from build123d import *

# Parameters (mm, degrees)
PAD015_DEPTH       = 15
SKETCH034_R        = 2
POCKET016_DEPTH    = 9.501
SKETCH_W           = 19.6
SKETCH_H           = 18.5
SKETCH_R           = 7.6
PAD_DEPTH          = 22
SKETCH002_W        = 17.1
SKETCH002_H        = 8.4
PAD001_DEPTH       = 8.5
POCKET_DEPTH       = 8
PAD002_DEPTH       = 13.6
SKETCH005_R        = 2
POCKET001_DEPTH    = 22.001
POCKET002_DEPTH    = 101.929968
POLARPATTERN_COUNT = 8
PAD004_DEPTH       = 1.5
SKETCH041_R        = 1.3
POCKET020_DEPTH    = 5


with BuildPart() as body026:
    # Sketch033 (on DatumPlane) → Pad015 (new body)
    with BuildSketch(Plane(origin=(0, -9.8, 0), x_dir=(0, 0, 1), z_dir=(0, -1, 0))):
        with BuildLine():
            Line((-9.5, 0), (-0.25, 0))
            Line((-0.25, 0), (-0.25, 6.907629))
            ThreePointArc((-0.25, 15.092371), (-4.1, 11), (-0.25, 6.907629))
            Line((-0.25, 15.092371), (-0.25, 22))
            Line((-0.25, 22), (-9.5, 22))
            Line((-9.5, 22), (-9.5, 0))
        make_face()
    extrude(amount=PAD015_DEPTH)

    # Sketch034 → Pocket016 (cut, through all)
    with BuildSketch(Plane.XY):
        with Locations((-18.546185, -13.8)):
            Circle(SKETCH034_R)
        with Locations((-3.453815, -13.8)):
            Circle(SKETCH034_R)
        with Locations((-3.453815, -20.8)):
            Circle(SKETCH034_R)
        with Locations((-18.546185, -20.8)):
            Circle(SKETCH034_R)
    extrude(amount=-POCKET016_DEPTH, mode=Mode.SUBTRACT)


with BuildPart() as printable_axisholder_y_fusion:
    # Sketch → Pad (new body)
    with BuildSketch(Plane.YZ):
        with Locations((0, -0.25)):
            Rectangle(SKETCH_W, SKETCH_H)
        Circle(SKETCH_R, mode=Mode.SUBTRACT)
    extrude(amount=-PAD_DEPTH)

    # Sketch002 → Pad001 (join)
    with BuildSketch(Plane(origin=(0, 0, 9), x_dir=(0, -1, 0), z_dir=(0, 0, 1))):
        with Locations((-1.25, -17.8)):
            Rectangle(SKETCH002_W, SKETCH002_H)
    extrude(amount=PAD001_DEPTH)

    # Sketch003 → Pocket (cut)
    with BuildSketch(Plane(origin=(0, -7.3, 0), x_dir=(0, 0, -1), z_dir=(0, -1, 0))):
        with BuildLine():
            Line((-10.5, -22), (-10.5, -13.6))
            Line((-10.5, -13.6), (-11.6, -13.6))
            ThreePointArc((-12.1, -14.1), (-11.746447, -13.953553), (-11.6, -13.6))
            ThreePointArc((-12.1, -14.1), (-12.6, -14.6), (-12.1, -15.1))
            ThreePointArc((-12.1, -16.1), (-11.6, -15.6), (-12.1, -15.1))
            ThreePointArc((-12.1, -16.1), (-12.6, -16.6), (-12.1, -17.1))
            ThreePointArc((-12.1, -18.1), (-11.6, -17.6), (-12.1, -17.1))
            ThreePointArc((-12.1, -18.1), (-12.6, -18.6), (-12.1, -19.1))
            ThreePointArc((-12.1, -20.1), (-11.6, -19.6), (-12.1, -19.1))
            ThreePointArc((-12.1, -20.1), (-12.6, -20.6), (-12.1, -21.1))
            ThreePointArc((-11.8, -22), (-11.625658, -21.441886), (-12.1, -21.1))
            Line((-11.8, -22), (-10.5, -22))
        make_face()
    extrude(amount=-POCKET_DEPTH, mode=Mode.SUBTRACT)

    # Sketch004 (on DatumPlane) → Pad002 (join)
    with BuildSketch(Plane.YZ):
        Polygon((9.8, 17.5), (1.3, 17.5), (1.3, 16.25), (8.55, 16.25), (8.55, 9), (9.8, 9), align=None)
    extrude(amount=-PAD002_DEPTH)

    # Sketch005 (on DatumPlane) → Pocket001 (cut, through all)
    with BuildSketch(Plane.YZ):
        with Locations((4, 12.625)):
            Circle(SKETCH005_R)
    extrude(amount=-POCKET001_DEPTH, mode=Mode.SUBTRACT)

    # Sketch006 (on DatumPlane) → Pocket002 (cut, through all)
    with BuildSketch(Plane.YZ):
        with BuildLine():
            ThreePointArc((-7.846282, 1.560723), (-8, 0), (-7.846282, -1.560723))
            Line((-6.708571, -1.334418), (-7.846282, -1.560723))
            ThreePointArc((-6.708571, 1.334418), (-6.84, 0), (-6.708571, -1.334418))
            Line((-6.708571, 1.334418), (-7.846282, 1.560723))
        make_face()
    pocket002 = extrude(amount=-POCKET002_DEPTH, mode=Mode.SUBTRACT)

    # PolarPattern: Pocket002 ×8 about axis
    polarpattern_axis = Axis((0, 0, 0), (1, 0, 0))
    for i in range(1, POLARPATTERN_COUNT):
        add(pocket002.rotate(polarpattern_axis, i * 360 / POLARPATTERN_COUNT), mode=Mode.SUBTRACT)

    # Sketch010 (on DatumPlane) → Pad004 (join)
    with BuildSketch(Plane.XY.offset(9)):
        Polygon((0, -7.8), (-13.6, -7.8), (-13.6, -7.3), (-22, -7.3), (-22, -9.8), (0, -9.8), align=None)
    extrude(amount=PAD004_DEPTH)

    # Sketch041 → Pocket020 (cut)
    with BuildSketch(Plane.XY.offset(-9.5)):
        with Locations((-11, 0)):
            Circle(SKETCH041_R)
    extrude(amount=POCKET020_DEPTH, mode=Mode.SUBTRACT)

    # Fusion001: union Body026
    add(body026.part)


solid = printable_axisholder_y_fusion.part
Source: CAD feature listing. Evaluate the final solid. Frame: model axes, mm. A direction names the side the tool comes from. Round coordinates to 2 decimals unless told otherwise and drop trailing zeros. Loops run counter-clockwise (first coordinate to the right, second up) from the corner with the lowest first, then second, coordinate; pieces in that order, holes last.
Q1. Mould query, pull axis Z, two halves, no side actions, for faces 1 (the face through (-18, -17, -0.25)), 2 (the face through (-16.64, -13.2, -4.81)), 3 (the face through (-10.846, 2.928, 7.013)). Classes: pulls with the +Z half, pulls with the -Z half, needs draft (parallel to the pull), parting line crosses it, or undercut.
Q2. Access query for faces 4 (the face through (-10.846, 7.013, -2.928)), 5 (the face through (-18, 0.7, 11)), 6 (the face through (-7, 8.55, 13)). Directions: +Z, -Z, +X, -X, +Y, -Y. A direction counts if a zero-diameter tool reaches every point of the face in a straight line with its end or side. Return the directions, or none.
Q3. Section D-D, the plane z = 3. Return loops of the section in (x, y).
Q4. Ray query, line 1 (Z direction, x = -17, y = 4) (3 decimals); line 2 (Y direction, x = -19, z = -5.75); line 3 (Z direction, x = -15, y = 7). Return the intervals inside material, ascending.
Q5. Section B-B, the plane z = -2. Return loops of the section in (x, y), plus the area to 3 significant figures.
Q6. First-contact query: P1, Ø3, axis at x = -6.5, y = -2.5, coming from the +Z side; P2, Ø3.5, axis at x = -2, y = -18.5, coming from the +Z side; P3, Ø0.6, axis at x = -18.5, z = 11, coming from the -Y side; P4, Ø8, axis at y = -11, z = 0, coming from the +X side. Flat tips, straight axial feed; report the tip coordinate or a pass-through.
Q7. Section A-A, the plane y = 0. Return loops of the section in (x, z).
Q8. Section C-C, the plane y = -13.8. Return loops of the section in (x, z), plus the area to 3 significant figures.
Solutions:
1. face 1: pulls with the +Z half
1. face 2: needs draft
1. face 3: undercut
2. face 4: +X, -X
2. face 5: -Y
2. face 6: +X
3. outline: (-22, -9.8) - (0, -9.8) - (0, -6.98) - (-22, -6.98) - close; (-22, 6.98) - (0, 6.98) - (0, 9.8) - (-22, 9.8) - close
4. line 1: z = -9.5 to -6.462, 6.462 to 10.625, 14.625 to 17.5
4. line 2: y = -24.8 to -22.75, -18.85 to -15.75, -11.85 to -5.56, 5.56 to 9.8
4. line 3: z = -9.5 to -2.96, 2.96 to 17.5
5. outline: (-22, -24.8) - (-14.58, -24.8) - (-14.58, -9.8) - (-7.42, -9.8) - (-7.42, -24.8) - (0, -24.8) - (0, -7.33) - (-22, -7.33) - close; (-22, 7.33) - (0, 7.33) - (0, 9.8) - (-22, 9.8) - close; hole circle Ø4 at (-18.55, -20.8); hole circle Ø4 at (-18.55, -13.8); hole circle Ø4 at (-3.45, -20.8); hole circle Ø4 at (-3.45, -13.8)
5. area: 281 mm2
6. P1: stops at z = 9
6. P2: stops at z = -0.25
6. P3: stops at y = 0.7
6. P4: stops at x = 0
7. outline: (-22, -9.5) - (-12.3, -9.5) - (-12.3, -8) - (-22, -8) - close; (-22, 8) - (0, 8) - (0, 9) - (-13.6, 9) - (-13.6, 10.5) - (-22, 10.5) - close; (-22, 11.8) arc R0.5 ccw to (-21.1, 12.1) arc R0.5 cw to (-20.1, 12.1) arc R0.5 ccw to (-19.1, 12.1) arc R0.5 cw to (-18.1, 12.1) arc R0.5 ccw to (-17.1, 12.1) arc R0.5 cw to (-16.1, 12.1) arc R0.5 ccw to (-15.1, 12.1) arc R0.5 cw to (-14.1, 12.1) arc R0.5 ccw to (-13.6, 11.6) - (-13.6, 17.5) - (-22, 17.5) - close; (-9.7, -9.5) - (0, -9.5) - (0, -8) - (-9.7, -8) - close
8. outline: (-22, -9.5) - (-20.55, -9.5) - (-20.55, -0.25) - (-22, -0.25) - close; (-16.55, -9.5) - (-5.45, -9.5) - (-5.45, -0.25) - (-6.91, -0.25) arc R4.1 cw to (-15.09, -0.25) - (-16.55, -0.25) - close; (-1.45, -9.5) - (0, -9.5) - (0, -0.25) - (-1.45, -0.25) - close
8. area: 105 mm2
